Build history of the part. All positions in model axes, mm. A direction names the side the tool comes from. Give positions to 0.01 mm unless a question says otherwise; leave off trailing zeros. Loops run counter-clockwise (first coordinate to the right, second up) from the corner with the lowest first, then second, coordinate; pieces in that order, holes last. Notation, with made-up numbers: (26.5, 33.25) -> (53.5, 33.25) arc R32 cw to (53.5, 61.25) -> close; hole circle Ø9 at (15.25, 82). An arc over 180 degrees is marked (long way). Answer as a JSON object with one key per item and string values. Group by question number.
Q1. Band-saw the part on A-A, the plane y = 11. Write the cut outline in (x, z).
Q2. Two-plate mould, pull along Y, no slides. Class faces 1 (the cylindrical face through (61.288, -175.863, 59.86)), 2 (the flat face through (-32, 2.968, 32)), 3 (the flat face through (43.408, -22, 25)): pulls with the +Y half, pulls with the -Y half, needs draft (parallel to the pull), parting line crosses it, or undercut.
Q3. Tool access for faces 4 (the flat face through (-45, -254, 30)), 5 (the cylindrical face through (-152.201, 136.006, 59.86)), 6 (the cylindrical face through (151.93, -93.54, 7.4)): list every direction of +Z, -Z, +X, -X, +Y, -Y with a clear straight run to the whole face (end or side of a thin tool).
Q4. Wall check: probe 1 along Z at (x, y) = (-18, 177.5); probe 2 along Z at (x, y) = (97, -162.5); probe 3 along Y at (x, z) = (-52, 31). Give the ranges that are in metal, low to high. Write a range as from..to.
Q5. Drop flat-ended pins along their axis: pin 1 (5.5 mm diameter, centred on x = -63, z = 31.5, fed in from +Y); pin 2 (14.5 mm diameter, centred on x = -21.15, z = 24.76, fed in from -Y); pin 3 (1.5 mm diameter, centred on x = -174, y = -215, fed in from +Z). Give the stop position or say it passes through.
Q6. Band-saw the part on B-B, the plane x = 137.5. Write the cut outline in (y, z), plus the area to 3 significant figures.
Q7. Band-saw the part on D-D, the plane y = -231. Write the cut outline in (x, z).
Q8. Band-saw the part on C-C, the plane y = 69. Write the cut outline in (x, z), plus the area to 3 significant figures.
from build123d import *

# Parameters (mm, degrees)
SKETCH1_R           = 200
BOSS_EXTRUDE1_DEPTH = 15
SKETCH2_W           = 148.705267073
SKETCH2_H           = 49.968568036
BOSS_EXTRUDE2_DEPTH = 20
CUT_EXTRUDE2_DEPTH  = 103
SKETCH4_R           = 280
BOSS_EXTRUDE3_DEPTH = 15
SKETCH6_R           = 40
BOSS_EXTRUDE4_DEPTH = 20
CIRPATTERN1_COUNT   = 4
SKETCH7_W           = 152.434020428
SKETCH7_H           = 72.590976785
BOSS_EXTRUDE5_DEPTH = 5


with BuildPart() as part:
    # Sketch1 → Boss-Extrude1 (new body)
    with BuildSketch(Plane.XY):
        with Locations((-32.819152061, -16.939919955)):
            Circle(SKETCH1_R)
    extrude(amount=BOSS_EXTRUDE1_DEPTH)

    # Sketch2 → Boss-Extrude2 (add)
    with BuildSketch(Plane.XY.offset(15)):
        with Locations((-30.944542613, -22.016117064)):
            Rectangle(SKETCH2_W, SKETCH2_H)
    extrude(amount=BOSS_EXTRUDE2_DEPTH)

    # Sketch3 → Cut-Extrude2 (cut)
    with BuildSketch(Plane(origin=(0, 2.968166954, 0), x_dir=(1, 0, 0), z_dir=(0, 1, 0))):
        with BuildLine():
            ThreePointArc((-28.877479091, -22.677000866), (-44.602439558, -24.756660882), (-28.877479091, -26.836320898))
            ThreePointArc((-28.877479091, -26.836320898), (-13.152518624, -24.756660882), (-28.877479091, -22.677000866))
        make_face()
    extrude(amount=-CUT_EXTRUDE2_DEPTH, mode=Mode.SUBTRACT)

    # Sketch4 → Boss-Extrude3 (add)
    with BuildSketch(Plane.XY.offset(35)):
        with Locations((-32.819152061, -25.168448638)):
            Circle(SKETCH4_R)
    extrude(amount=BOSS_EXTRUDE3_DEPTH)

    # Sketch6 → Boss-Extrude4 (add)
    with BuildSketch(Plane.XY.offset(50)):
        with Locations((-154.032312031, -146.309301386)):
            Circle(SKETCH6_R)
    boss_extrude4 = extrude(amount=BOSS_EXTRUDE4_DEPTH)

    # CirPattern1: Boss-Extrude4 ×4 about axis
    cirpattern1_axis = Axis((-32.819152061, -25.168448638, 0), (0, 0, 1))
    for i in range(1, CIRPATTERN1_COUNT):
        add(boss_extrude4.rotate(cirpattern1_axis, i * 360 / CIRPATTERN1_COUNT))

    # Sketch7 → Boss-Extrude5 (add)
    with BuildSketch(Plane(origin=(0, 0, 35), x_dir=(-1, 0, 0), z_dir=(0, 0, -1))):
        with Locations((46.178823142, -254.15774716)):
            Rectangle(SKETCH7_W, SKETCH7_H)
    extrude(amount=BOSS_EXTRUDE5_DEPTH)


solid = part.part
Worked answers:
{
 "1": {"outline": "(-310.47, 35) -> (244.84, 35) -> (244.84, 50) -> (-310.47, 50) -> close; (-230.86, 0) -> (165.22, 0) -> (165.22, 15) -> (-230.86, 15) -> close"},
 "2": {"face 1": "undercut", "face 2": "pulls with the +Y half", "face 3": "needs draft"},
 "3": {"face 4": "-Z, +X, -X, -Y", "face 5": "+Z", "face 6": "-Z"},
 "4": {"probe 1": "0..15, 35..50", "probe 2": "0..15, 35..70", "probe 3": "-290.45..-217.86, -47..2.97"},
 "5": {"pin 1": "y = 2.97", "pin 2": "y = -290.45", "pin 3": "z = 50"},
 "6": {"outline": "(-247.41, 35) -> (197.07, 35) -> (197.07, 50) -> (-247.41, 50) -> close; (-121.78, 0) -> (87.9, 0) -> (87.9, 15) -> (-121.78, 15) -> close", "area": "9,810 mm2"},
 "7": {"outline": "(-222.64, 35) -> (-122.4, 35) -> (-122.4, 30) -> (30.04, 30) -> (30.04, 35) -> (157.01, 35) -> (157.01, 50) -> (-222.64, 50) -> close"},
 "8": {"outline": "(-296.51, 35) -> (230.87, 35) -> (230.87, 50) -> (117.93, 50) -> (117.93, 70) -> (58.86, 70) -> (58.86, 50) -> (-124.49, 50) -> (-124.49, 70) -> (-183.43, 70) -> (-183.43, 50) -> (-296.51, 50) -> close; (-213.41, 0) -> (147.78, 0) -> (147.78, 15) -> (-213.41, 15) -> close", "area": "15,700 mm2"}
}
